```python
from build123d import *

# Parameters (mm, degrees)
SKETCH_1_W           = 90
SKETCH_1_H           = 58
EXTRUDE_1_DEPTH      = 3
SKETCH_3_OUTSIDE_W   = 113.422
SKETCH_3_OUTSIDE_H   = 81.422
SKETCH_3_OUTSIDE_W_2 = 3
SKETCH_3_OUTSIDE_H_2 = 34
CUT_EXTRUDE_1_DEPTH  = 3
SKETCH_4_W           = 9
SKETCH_4_H           = 30
CUT_EXTRUDE_2_DEPTH  = 4
FILLET_1_R           = 3
EXTRUDE_2_DEPTH      = 3


with BuildPart() as part:
    # 스케치1 → 보스-돌출1 (new body)
    with BuildSketch(Plane(origin=(0, 0, 0), x_dir=(0, 0, -1), z_dir=(1, 0, 0))):
        with Locations((45, 29)):
            Rectangle(SKETCH_1_W, SKETCH_1_H)
    extrude(amount=EXTRUDE_1_DEPTH)

    # 스케치3 outside → 컷-돌출1 (cut)
    with BuildSketch(Plane(origin=(3, 0, 0), x_dir=(0, 0, -1), z_dir=(1, 0, 0))):
        with Locations((45, 29)):
            Rectangle(SKETCH_3_OUTSIDE_W, SKETCH_3_OUTSIDE_H)
        Polygon((44.864431473, 50), (56.362384973, 50), (56.362384973, 58), (72.348389068, 58), (72.348389068, 50), (89.728862946, 50), (89.728862946, 8), (72.348389068, 8), (72.348389068, 0), (56.362384973, 0), (56.362384973, 8), (44.864431473, 8), (0, 15.482252367), (0, 42.517747633), align=None, mode=Mode.SUBTRACT)
        with Locations((82.5, 29)):
            Rectangle(SKETCH_3_OUTSIDE_W_2, SKETCH_3_OUTSIDE_H_2)
    extrude(amount=-CUT_EXTRUDE_1_DEPTH, mode=Mode.SUBTRACT)

    # 스케치4 → 컷-돌출2 (cut, through all)
    with BuildSketch(Plane(origin=(3, 0, 0), x_dir=(0, 0, -1), z_dir=(1, 0, 0))):
        with Locations((69.481068703, 29)):
            Rectangle(SKETCH_4_W, SKETCH_4_H)
    extrude(amount=-CUT_EXTRUDE_2_DEPTH, mode=Mode.SUBTRACT)

    # 필렛1
    fillet_1_edges = [part.edges().sort_by_distance(p)[0] for p in [
        (1.5, 8, -72.348389068),
        (1.5, 0, -72.348389068),
        (1.5, 0, -56.362384973),
        (1.5, 8, -56.362384973),
        (1.5, 8, -44.864431473),
        (1.5, 15.482252367, 0),
        (1.5, 42.517747633, 0),
        (1.5, 50, -44.864431473),
        (1.5, 50, -56.362384973),
        (1.5, 58, -56.362384973),
        (1.5, 58, -72.348389068),
    ]]
    fillet(fillet_1_edges, radius=FILLET_1_R)

    # 스케치5 → 보스-돌출2 (add)
    with BuildSketch(Plane(origin=(3, 0, 0), x_dir=(0, 0, -1), z_dir=(1, 0, 0))):
        Polygon((84, 43), (83.133974596, 42.5), (84, 42), align=None)
        Polygon((83.133974596, 15.5), (84, 16), (84, 15), align=None)
    extrude(amount=-EXTRUDE_2_DEPTH)


solid = part.part
```
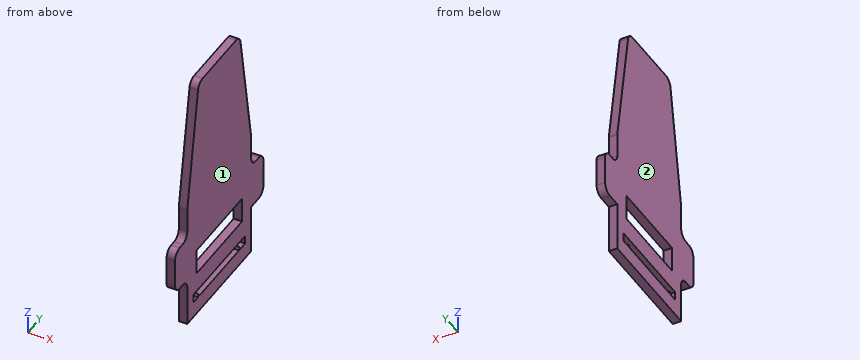
The listing builds one solid part. Answer for the finished solid, in the listing's coordinates (mm). Face numbers are marked on the shaded views. Give positions to 0.01 mm unless a question says otherwise; leave off trailing zeros. Loops run counter-clockwise (first coordinate to the right, second up) from the corner with the lowest first, then second, coordinate; pieces in that order, holes last. Notation, with made-up numbers: (54.5, 15.5) - (82.5, 15.5) arc R22 cw to (82.5, 54.5) - close; hole circle Ø7 at (-33, 68.25). An arc over 180 degrees is marked (long way). Answer as CSV lines item,"result". Start each with the question number.
Item 1: Find the intervals of material crossed by line 1 (Z direction, x = 2.25, y = 19); line 2 (Y direction, x = 1.45, z = -82); line 3 (Z direction, x = 1.7, y = 42), in increasing order. Write a range as from..to.
Item 2: Each of these flat-tipped pins is pushed along its axis until it touches: pin 1 (12 mm diameter, centred on y = 32, z = -46, fed in from -X); pin 2 (1.5 mm diameter, centred on x = 2, z = -85.5, fed in from -Y); pin 3 (0.6 mm diameter, centred on x = 1.5, y = 3.5, fed in from -Z); pin 4 (1.5 mm diameter, centred on x = 1.5, z = -82.5, fed in from +Y). Where does it stop, or does it pass through?
Item 3: A cutting plane is placed at D-D on z = -39.5. Determine the outline of the cut face in (x, y), then the cut area to 3 significant figures.
Item 4: A cutting plane is placed at C-C on x = 0.75. Count the separate pieces of the cut face and the enclosed holes in it, then the cut area to 3 significant figures.
Item 5: A cutting plane is placed at A-A on y = 22.5. Determine the outline of the cut face in (x, z), then the cut area to 3 significant figures.
Item 6: The mould has two halves that part along X. Classify the marked faces 1 and 2: +X half, -X half, draft (parallel to the pull), parting line (faces both ways), or undercut.
Item 7: A cutting plane is placed at B-B on z = -71. Determine the outline of the cut face in (x, y).
Found:
1,line 1,"z = -89.73..-84, -81..-73.98, -64.98..0"
1,line 2,"y = 8..12, 46..50"
1,line 3,"z = -89.73..-84, -81..-73.98, -64.98..-0.79"
2,pin 1,"stops at x = 0"
2,pin 2,"stops at y = 8"
2,pin 3,"stops at z = -72.35"
2,pin 4,"stops at y = 50"
3,outline,"(0, 8.89) - (3, 8.89) - (3, 49.11) - (0, 49.11) - close"
3,area,"121 mm^2"
4,separate pieces,"1"
4,enclosed holes,"2"
4,area,"3,310 mm^2"
5,outline,"(0, -89.73) - (3, -89.73) - (3, -84) - (0, -84) - close; (0, -81) - (3, -81) - (3, -73.98) - (0, -73.98) - close; (0, -64.98) - (3, -64.98) - (3, 0) - (0, 0) - close"
5,area,"233 mm^2"
6,face 1,"+X half"
6,face 2,"-X half"
7,outline,"(0, 0.5) - (3, 0.5) - (3, 14) - (0, 14) - close; (0, 44) - (3, 44) - (3, 57.5) - (0, 57.5) - close"
